from build123d import *

# Parameters (mm, degrees)
SKETCH3_W           = 70
SKETCH3_H           = 70
SKETCH3_R           = 3
BOSS_EXTRUDE2_DEPTH = 3
FILLET2_R           = 3


with BuildPart() as part:
    # Sketch3 → Boss-Extrude2 (new body)
    with BuildSketch(Plane.XY):
        Rectangle(SKETCH3_W, SKETCH3_H)
        with Locations((0, 10)):
            Circle(SKETCH3_R, mode=Mode.SUBTRACT)
        with Locations((-24.3, 24.3)):
            Circle(SKETCH3_R, mode=Mode.SUBTRACT)
        with Locations((10, 0)):
            Circle(SKETCH3_R, mode=Mode.SUBTRACT)
        with Locations((0, -10)):
            Circle(SKETCH3_R, mode=Mode.SUBTRACT)
        with Locations((-10, 0)):
            Circle(SKETCH3_R, mode=Mode.SUBTRACT)
        with Locations((-24.3, -24.3)):
            Circle(SKETCH3_R, mode=Mode.SUBTRACT)
        with Locations((24.3, 0)):
            Circle(SKETCH3_R, mode=Mode.SUBTRACT)
    extrude(amount=BOSS_EXTRUDE2_DEPTH)

    # Fillet2
    fillet2_edges = [part.edges().sort_by_distance(p)[0] for p in [
        (35, -35, 1.5),
        (-35, -35, 1.5),
        (-35, 35, 1.5),
        (35, 35, 1.5),
    ]]
    fillet(fillet2_edges, radius=FILLET2_R)


solid = part.part
Check sheet for the modelled part. Datum: model origin and axes. Units: mm. Give positions to 0.01 mm unless a question says otherwise; leave off trailing zeros. Loops run counter-clockwise (first coordinate to the right, second up) from the corner with the lowest first, then second, coordinate; pieces in that order, holes last. Notation, with made-up numbers: M -29.75,67 L 15.25,67 A22 cw 15.25,84 Z; hole C 82.5,-2 d10. An arc over 180 degrees is marked long. Answer as a JSON object with one key per item and string values. Group by question number.
Q1. Go/stop test with a flat-tipped pin: P1, Ø9.5, axis at x = 24.3, y = 0, coming from the +Z side. Record where the tip stops, or that it passes through.
Q2. Release check for a two-part mould opening along X. For faces 1 (the flat face through (0, 0, 3)), 2 (the cylindrical face through (-24.95, 21.37, 1.48)), 3 (the cylindrical face through (-34.14, -34.1, 1.52)) record: released by +X, released by -X, zero draft, split by the parting line, or undercut.
Q3. Material ranges on line 1 along Y through (x, z) = (0, 2.2); line 2 along Y through (x, z) = (-24.3, 1.5); line 3 along Y through (x, z) = (10, 1.65), recorded low to high. Write a range as [from, to].
Q4. Cross-section at A-A on x = -24.3. Record the cut outline in (y, z).
Q5. Cross-section at B-B on y = 10. Record the cut outline in (x, z), then the cut area to 3 significant figures.
Q6. Cross-section at C-C on z = 1. Record the cut outline in (x, y), then the cut area to 3 significant figures.
Evaluation:
{
 "1": {"P1": "stops at z = 3"},
 "2": {"face 1": "zero draft", "face 2": "undercut", "face 3": "released by -X"},
 "3": {"line 1": "y = [-35, -13], [-7, 7], [13, 35]", "line 2": "y = [-35, -27.3], [-21.3, 21.3], [27.3, 35]", "line 3": "y = [-35, -3], [3, 35]"},
 "4": {"outline": "M -35,0 L -27.3,0 L -27.3,3 L -35,3 Z; M -21.3,0 L 21.3,0 L 21.3,3 L -21.3,3 Z; M 27.3,0 L 35,0 L 35,3 L 27.3,3 Z"},
 "5": {"outline": "M -35,0 L -3,0 L -3,3 L -35,3 Z; M 3,0 L 35,0 L 35,3 L 3,3 Z", "area": "192 mm2"},
 "6": {"outline": "M -35,-32 A3 ccw -32,-35 L 32,-35 A3 ccw 35,-32 L 35,32 A3 ccw 32,35 L -32,35 A3 ccw -35,32 Z; hole C -24.3,-24.3 d6; hole C -24.3,24.3 d6; hole C -10,0 d6; hole C 0,-10 d6; hole C 0,10 d6; hole C 10,0 d6; hole C 24.3,0 d6", "area": "4,690 mm2"}
}
